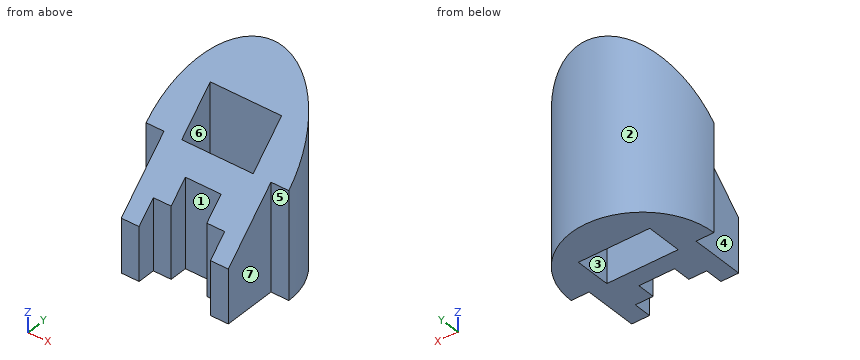
```python
from build123d import *

# Parameters (mm, degrees)
SKETCH2_W           = 4
SKETCH2_H           = 2
BOSS_EXTRUDE1_DEPTH = 5
CUT_EXTRUDE1_DEPTH  = 4


with BuildPart() as part:
    # Sketch2 → Boss-Extrude1 (new body, symmetric)
    with BuildSketch(Plane.XY):
        with BuildLine():
            Line((-4, -1), (-3, -1))
            Line((-3, -1), (-3, -4))
            Line((-3, -4), (-2, -4))
            Line((-2, -4), (-2, -3))
            Line((-2, -3), (-1, -3))
            Line((-1, -3), (-1, -2))
            Line((-1, -2), (1, -2))
            Line((1, -2), (1, -3))
            Line((1, -3), (2, -3))
            Line((2, -3), (2, -4))
            Line((2, -4), (3, -4))
            Line((3, -4), (3, -1))
            Line((3, -1), (4, -1))
            ThreePointArc((4, -1), (0, 3), (-4, -1))
        make_face()
        Rectangle(SKETCH2_W, SKETCH2_H, mode=Mode.SUBTRACT)
    extrude(amount=BOSS_EXTRUDE1_DEPTH, both=True)

    # Sketch3 → Cut-Extrude1 (cut, symmetric)
    with BuildSketch(Plane(origin=(0, 0, 0), x_dir=(0, 0, -1), z_dir=(1, 0, 0))):
        Polygon((-5, 3), (2, -4), (-5, -4), align=None)
    extrude(amount=CUT_EXTRUDE1_DEPTH, both=True, mode=Mode.SUBTRACT)


solid = part.part
```
Here's how the part is built. I have some questions about the finished solid (model axes, mm). Face numbers are marked on the shaded views. A direction names the side the tool comes from. Round coordinates to 2 decimals unless told otherwise and drop trailing zeros. Order: outer loops, then holes, each group sorted by start corner. A loop starts at its lowest first (then second) coordinate and runs counter-clockwise, first axis right, second up. Notation, with made-up numbers: M 33,-10 L 62,-10 A21 ccw 62,29 Z; hole C 19.5,-7.75 d9. An arc over 180 degrees is marked long. One line per question, with ' | ' between items.
1) I want a section at C-C, the plane z = 0.75. Write out the boundary of the cut face in (x, y).
Working result:
outline: M -4,-1 L -3,-1 L -3,-1.25 L 3,-1.25 L 3,-1 L 4,-1 A4 ccw Z; hole M -2,-1 L 2,-1 L 2,1 L -2,1 Z
2) I want a section at D-D, the plane z = -0.25. Write out the boundary of the cut face in (x, y), then the cut area to 3 significant figures.
Working result:
outline: M -4,-1 L -3,-1 L -3,-2.25 L -1,-2.25 L -1,-2 L 1,-2 L 1,-2.25 L 3,-2.25 L 3,-1 L 4,-1 A4 ccw Z; hole M -2,-1 L 2,-1 L 2,1 L -2,1 Z | area: 24.1 mm²
3) If we mould it in two halves opening along X, with no side actions, what happens to the marked faces 5, 6 and 7? For each: +X half, -X half, draft (parallel to the pull), parting line (faces both ways), or undercut.
Working result:
face 5: draft | face 6: undercut | face 7: +X half
4) I need wall thicknesses on line 1 along X through (y, z) = (-2.75, -3.5); line 2 along X through (y, z) = (-3.5, -3.5); line 3 along Y through (x, z) = (-0.75, -4.5). Which ranges of each line are inside material? Lowest first, please.
Working result:
line 1: -3 to -1, 1 to 3 | line 2: -3 to -2, 2 to 3 | line 3: -2 to -1, 1 to 2.93
5) For pin 1 Ø0.5 at (y, z) = (-3.5, -4) entering from +X; pin 2 Ø2 at (x, z) = (0.5, -2) entering from +Y; pin 3 Ø2 at (x, y) = (2, -1.5) entering from +Z; pin 4 Ø0.5 at (x, z) = (-3.5, -0.5) entering from -Y, each with a flat end and sliding along its axis, tell me the tip position at first contact or that it passes through.
Working result:
pin 1: x = 3 | pin 2: y = 3 | pin 3: z = 1.5 | pin 4: y = -1
6) For the marked faces 1, 2, 3 and 4, which set-ups out of +Z, -Z, +X, -X, +Y, -Y let a thin tool reach every point of the face, with its end or its side?
Working result:
face 1: +Z, -Z, -Y | face 2: +Z, -Z, +Y | face 3: +Z, -Z | face 4: +Z, -Z, -X, -Y
7) I want a section at B-B, the plane x = 0. Write out the boundary of the cut face in (y, z), then the cut area to 3 significant figures.
Working result:
outline: M -2,-5 L -1,-5 L -1,1 L -2,0 Z; M 1,-5 L 3,-5 L 3,5 L 1,3 Z | area: 23.5 mm²
8) I want a section at A-A, the plane y = -3.5. Write out the boundary of the cut face in (x, z).
Working result:
outline: M -3,-5 L -2,-5 L -2,-1.5 L -3,-1.5 Z; M 2,-5 L 3,-5 L 3,-1.5 L 2,-1.5 Z
